from build123d import *

# Parameters (mm, degrees)
SKETCH_R             = 3.1
PAD_DEPTH            = 13
SKETCH001_R          = 2.6
POCKET_DEPTH         = 11
POCKET001_DEPTH      = 8.5
POCKET002_DEPTH      = 13.001
POCKET002_DEPTH_BACK = -13.001
SKETCH004_W          = 18.821557
SKETCH004_H          = 5.678009
SKETCH004_H_2        = 5.407065
SKETCH004_W_2        = 10.052157
SKETCH004_H_3        = 19
POCKET003_DEPTH      = 6.501
POCKET003_DEPTH_BACK = -6.501
CHAMFER_SIZE         = 0.5
CHAMFER001_SIZE      = 0.35
CHAMFER002_SIZE      = 0.4
CHAMFER003_SIZE      = 1


with BuildPart() as part:
    # Sketch → Pad (new body, symmetric)
    with BuildSketch(Plane.XZ):
        with BuildLine():
            ThreePointArc((-6.5, 6.5), (-13, 0), (-6.5, -6.5))
            Line((-6.5, -6.5), (13, -6.5))
            Line((13, -6.5), (13, 0))
            ThreePointArc((13, 0), (12.932748, 0.682816), (12.733578, 1.339392))
            Line((10.595985, 6.5), (12.733578, 1.339392))
            Line((10.595985, 6.5), (-6.5, 6.5))
        make_face()
        with Locations((-6.5, 0)):
            Circle(SKETCH_R, mode=Mode.SUBTRACT)
    extrude(amount=PAD_DEPTH, both=True)

    # Sketch001 → Pocket (cut, symmetric)
    with BuildSketch(Plane.XZ):
        with BuildLine():
            ThreePointArc((3, 3.5), (2.117588, 0), (3, -3.5))
            Line((3, -3.5), (3, -7.382412))
            Line((3, -7.382412), (9.5, -7.382412))
            ThreePointArc((9.5, -7.382412), (16.882412, 0), (9.5, 7.382412))
            Line((9.5, 7.382412), (3, 7.382412))
            Line((3, 7.382412), (3, 3.5))
        make_face()
        with Locations((9.5, 0)):
            Circle(SKETCH001_R, mode=Mode.SUBTRACT)
    extrude(amount=POCKET_DEPTH, both=True, mode=Mode.SUBTRACT)

    # Sketch002 → Pocket001 (cut, symmetric)
    with BuildSketch(Plane.XZ):
        with BuildLine():
            Line((-3, 3.5), (3, 3.5))
            Line((3, 3.5), (3, -9.5))
            Line((3, -9.5), (14.967288, -9.5))
            Line((14.967288, -9.5), (14.967288, 9.5))
            Line((14.967288, 9.5), (-6.5, 9.5))
            ThreePointArc((-6.5, 9.5), (-16, 0), (-6.5, -9.5))
            Line((-3, -9.5), (-6.5, -9.5))
            Line((-3, 3.5), (-3, -9.5))
        make_face()
    extrude(amount=POCKET001_DEPTH, both=True, mode=Mode.SUBTRACT)

    # Sketch003 → Pocket002 (cut, two sides)
    with BuildSketch(Plane.YZ) as pocket002_sk:
        with BuildLine():
            Line((-7.5, 8.494664), (7.5, 8.494664))
            Line((7.5, 8.494664), (7.5, -1.5))
            ThreePointArc((5.5, -3.5), (6.914214, -2.914214), (7.5, -1.5))
            Line((5.5, -3.5), (-5.5, -3.5))
            ThreePointArc((-7.5, -1.5), (-6.914214, -2.914214), (-5.5, -3.5))
            Line((-7.5, -1.5), (-7.5, 8.494664))
        make_face()
    extrude(amount=-POCKET002_DEPTH, mode=Mode.SUBTRACT)
    extrude(pocket002_sk.sketch, amount=-POCKET002_DEPTH_BACK, mode=Mode.SUBTRACT)

    # Sketch004 → Pocket003 (cut, two sides)
    with BuildSketch(Plane.XY) as pocket003_sk:
        with Locations((-12.410778, 13.339004)):
            Rectangle(SKETCH004_W, SKETCH004_H)
        with Locations((-12.410778, -13.203532)):
            Rectangle(SKETCH004_W, SKETCH004_H_2)
        with Locations((10.204497, 0)):
            Rectangle(SKETCH004_W_2, SKETCH004_H_3)
    extrude(amount=-POCKET003_DEPTH, mode=Mode.SUBTRACT)
    extrude(pocket003_sk.sketch, amount=-POCKET003_DEPTH_BACK, mode=Mode.SUBTRACT)

    # Chamfer
    chamfer_edges = [part.edges().sort_by_distance(p)[0] for p in [
        (6.9, 9.5, 0),
        (6.9, -9.5, 0),
    ]]
    chamfer(chamfer_edges, length=CHAMFER_SIZE)

    # Chamfer001
    chamfer001_edges = [part.edges().sort_by_distance(p)[0] for p in [
        (6.9, 11, 0),
        (6.9, -11, 0),
    ]]
    chamfer(chamfer001_edges, length=CHAMFER001_SIZE)

    # Chamfer002
    chamfer002_edges = [part.edges().sort_by_distance(p)[0] for p in [
        (-9.6, -10.5, 0),
        (-9.6, 10.5, 0),
    ]]
    chamfer(chamfer002_edges, length=CHAMFER002_SIZE)

    # Chamfer003
    chamfer003_edges = [part.edges().sort_by_distance(p)[0] for p in [
        (3.797992, 13, 6.5),
        (5, 13, -6.5),
        (5, -13, -6.5),
        (3.797992, -13, 6.5),
    ]]
    chamfer(chamfer003_edges, length=CHAMFER003_SIZE)


solid = part.part
Work out the finished part from the listing and answer in its coordinate system (mm). A direction names the side the tool comes from. Give positions to 0.01 mm unless a question says otherwise; leave off trailing zeros. Loops run counter-clockwise (first coordinate to the right, second up) from the corner with the lowest first, then second, coordinate; pieces in that order, holes last. Notation, with made-up numbers: (73.25, -14.5) - (113.25, -14.5) arc R12 ccw to (113.25, 7.5) - close; hole circle Ø4 at (30, 30). An arc over 180 degrees is marked (long way). Answer in a Markdown table with one row per item.
(1) A tool of negligible diameter and unlimited length cuts with its end or side. For faces 4 (the face through (-5, 8.5, 3)), 5 (the face through (0, 0, -3.5)), 6 (the face through (-3, 12, 0)), 7 (the face through (6, -11, 0)), from which of +Z, -Z, +X, -X, +Y, -Y can it reach the whole face along a straight path? Write none if from no direction.
Results list:
| item | result |
|---|---|
| face 4 | +Z, -X |
| face 5 | +Z, +X, -X |
| face 6 | +Z, -Z, -X, +Y |
| face 7 | none |
(2) Section D-D (x = -7) is taken. State how many separate pieces and enclosed holes the cut face has, and give its area (3 significant figures).
Results list:
| item | result |
|---|---|
| separate pieces | 4 |
| enclosed holes | 0 |
| area | 27.0 mm² |
(3) Section C-C (x = 9.5) is taken. Give the vertices of the cut face in (y, z), and give its area (3 significant figures).
Results list:
| item | result |
|---|---|
| outline | (-13, -5.5) - (-12, -6.5) - (-11, -6.5) - (-11, -2.95) - (-10.65, -2.6) - (-10, -2.6) - (-9.5, -2.1) - (-9.5, 2.1) - (-10, 2.6) - (-10.65, 2.6) - (-11, 2.95) - (-11, 6.5) - (-12, 6.5) - (-13, 5.5) - close; (9.5, -2.1) - (10, -2.6) - (10.65, -2.6) - (11, -2.95) - (11, -6.5) - (12, -6.5) - (13, -5.5) - (13, 5.5) - (12, 6.5) - (11, 6.5) - (11, 2.95) - (10.65, 2.6) - (10, 2.6) - (9.5, 2.1) - close |
| area | 65.3 mm² |
(4) Section B-B (y = 9) is taken. Give the vertices of the cut face in (x, z).
Results list:
| item | result |
|---|---|
| outline | (-6.5, -6.5) - (3, -6.5) - (3, -3.5) arc R7.38 cw to (3, 3.5) - (3, 6.5) - (-6.5, 6.5) arc R6.5 ccw to start; hole circle Ø6.2 at (-6.5, 0) |
(5) Section A-A (x = 5.75) is taken. Give the vertices of the cut face in (y, z).
Results list:
| item | result |
|---|---|
| outline | (-13, -5.5) - (-12, -6.5) - (-11, -6.5) - (-11, 6.5) - (-12, 6.5) - (-13, 5.5) - close; (11, -6.5) - (12, -6.5) - (13, -5.5) - (13, 5.5) - (12, 6.5) - (11, 6.5) - close |
(6) Consider L1, parallel to Y at x = 8.5, z = 1; L2, parallel to Y at x = 9.25, z = 3.75; L3, parallel to Z at x = -6.5, y = -9.3. Determine where each line is inside the solid, lowest interval first. Write a range as [from, to].
Results list:
| item | result |
|---|---|
| L1 | y = [-13, -9.5], [9.5, 13] |
| L2 | y = [-13, -11], [11, 13] |
| L3 | z = [-6.5, -3.1], [3.1, 6.5] |
(7) For a pull along Y with two mould halves and no side action, classify faces 1 (the face through (-10.3, 10.5, 0.1)), 2 (the face through (11.98, 10.33, 0.78)), 3 (the face through (0, 10, 6.5)) as pulls with the +Y half, pulls with the -Y half, needs draft (parallel to the pull), parting line crosses it, or undercut.
Results list:
| item | result |
|---|---|
| face 1 | pulls with the +Y half |
| face 2 | undercut |
| face 3 | needs draft |
(8) Flat-ended cylindrical pins translate along their axes: pin 1 Ø2.5 at (y, z) = (-1.5, -4.5) entering from +X; pin 2 Ø5 at (x, z) = (-9.5, -3) entering from +Y; pin 3 Ø0.5 at (x, y) = (0.5, -8) entering from +Z. Find the tip coordinate at first contact, or state that the pin passes through.
Results list:
| item | result |
|---|---|
| pin 1 | stops at x = 3 |
| pin 2 | stops at y = 10.5 |
| pin 3 | stops at z = 3.5 |
